The model under review builds one solid part; all positions refer to its coordinate system, in mm. Coordinates: 2 decimals unless noted, no trailing zeros. Write each loop counter-clockwise with the first axis right and the second up, starting at its lowest first coordinate (ties: lowest second). Pieces come first, ordered by that corner, then holes. Notation, with made-up numbers: (79.25, -36.5) - (133.25, -36.5) arc R25 cw to (133.25, -10.5) - close; hole circle Ø4 at (-20, 62). An arc over 180 degrees is marked (long way). Put each result on its own line as item: value. Start each with the question number.
Item 1: Consider section C-C on x = 4. Give the boundary of the cut face in (y, z), then the cut area to 3 significant figures.
Item 2: Consider section B-B on z = 3.55. Give the boundary of the cut face in (x, y), then the cut area to 3 significant figures.
Item 3: Consider section A-A on y = 0. Give the boundary of the cut face in (x, z).
Item 4: To check wall thickness, follow L1, parallel to Z at x = -2.5, y = 1.05; L2, parallel to X at y = 1.35, z = 1.9; L3, parallel to X at y = -0.9, z = 3. State the ranges of each line that lie inside material, in increasing order. Write a range as [from, to].
Item 5: Mouldability with a two-part tool opening along Y and no side actions: class faces 1 (the face through (0, 0, 5.556)), 2 (the face through (3.06, 0.54, 3.14)) as pulls with the +Y half, pulls with the -Y half, needs draft (parallel to the pull), parting line crosses it, or undercut.
Item 6: Consider section D-D on y = -0.95. State how many separate pieces and enclosed holes the cut face has, then the cut area to 3 significant figures.
```python
from build123d import *

# Parameters (mm, degrees)
BOSS_EXTRUDE1_DEPTH = 1.5875
SKETCH2_R           = 3.175
BOSS_EXTRUDE2_DEPTH = 3.175
SKETCH3_R           = 2.38125
CUT_EXTRUDE1_DEPTH  = 6.35
SCALE1_SCALE        = 0.75


with BuildPart() as part:
    # Sketch1 → Boss-Extrude1 (new body)
    with BuildSketch(Plane.XY):
        with BuildLine():
            ThreePointArc((-4.10493597, 2.24506403), (-9.525, 0), (-4.10493597, -2.24506403))
            add(Edge.make_bspline(
                [(-4.10493597, -2.24506403), (0, 0.65756403), (4.10493597, -2.24506403)],
                knots=[0, 0, 0, 1, 1, 1], degree=2))
            ThreePointArc((4.10493597, -2.24506403), (9.525, 0), (4.10493597, 2.24506403))
            add(Edge.make_bspline(
                [(-4.10493597, 2.24506403), (0, -0.65756403), (4.10493597, 2.24506403)],
                knots=[0, 0, 0, 1, 1, 1], degree=2))
        make_face()
    boss_extrude1 = extrude(amount=BOSS_EXTRUDE1_DEPTH)

    # Sketch2 → Boss-Extrude2 (add)
    with BuildSketch(Plane.XY.offset(1.5875)):
        with Locations(Location((-6.35, 0, 0), (0, 0, 315))):
            Circle(SKETCH2_R)
        with Locations(Location((6.35, 0, 0), (0, 0, 135))):
            Circle(SKETCH2_R)
    extrude(amount=BOSS_EXTRUDE2_DEPTH)

    # Mirror1: Boss-Extrude1 across plane
    add(boss_extrude1.mirror(Plane.XY.offset(3.175)))

    # Sketch3 → Cut-Extrude1 (cut)
    with BuildSketch(Plane(origin=(0, 0, 0), x_dir=(-1, 0, 0), z_dir=(0, 0, -1))):
        with Locations((-6.35, 0)):
            Circle(SKETCH3_R)
        with Locations((6.35, 0)):
            Circle(SKETCH3_R)
    extrude(amount=-CUT_EXTRUDE1_DEPTH, mode=Mode.SUBTRACT)


with BuildPart() as part_1:
    # Scale1: scaled about (0, 0, 3.175)
    add(part.part.scale(SCALE1_SCALE).moved(Location((0, 0, 0.79375))))


solid = part_1.part
```
Report:
1. outline: (-2.26, 0.79) - (-1.61, 0.79) - (-1.61, 5.56) - (-2.26, 5.56) - close; (1.61, 0.79) - (2.26, 0.79) - (2.26, 5.56) - (1.61, 5.56) - close
1. area: 6.10 mm²
2. outline: circle Ø4.76 at (-4.76, 0); circle Ø4.76 at (4.76, 0); hole circle Ø3.57 at (-4.76, 0); hole circle Ø3.57 at (4.76, 0)
2. area: 15.6 mm²
3. outline: (-7.14, 0.79) - (-6.55, 0.79) - (-6.55, 5.56) - (-7.14, 5.56) - close; (-2.98, 0.79) - (2.98, 0.79) - (2.98, 5.56) - (-2.98, 5.56) - close; (6.55, 0.79) - (7.14, 0.79) - (7.14, 5.56) - (6.55, 5.56) - close; hole (-2.38, 1.98) - (2.38, 1.98) - (2.38, 4.37) - (-2.38, 4.37) - close
4. L1: [0.79, 1.98], [4.37, 5.56]
4. L2: [-6.72, -5.93], [-3.59, -2.56], [2.56, 3.59], [5.93, 6.72]
4. L3: [-6.97, -6.31], [-3.22, -2.56], [2.56, 3.22], [6.31, 6.97]
5. face 1: needs draft
5. face 2: undercut
6. separate pieces: 4
6. enclosed holes: 0
6. area: 16.7 mm²
